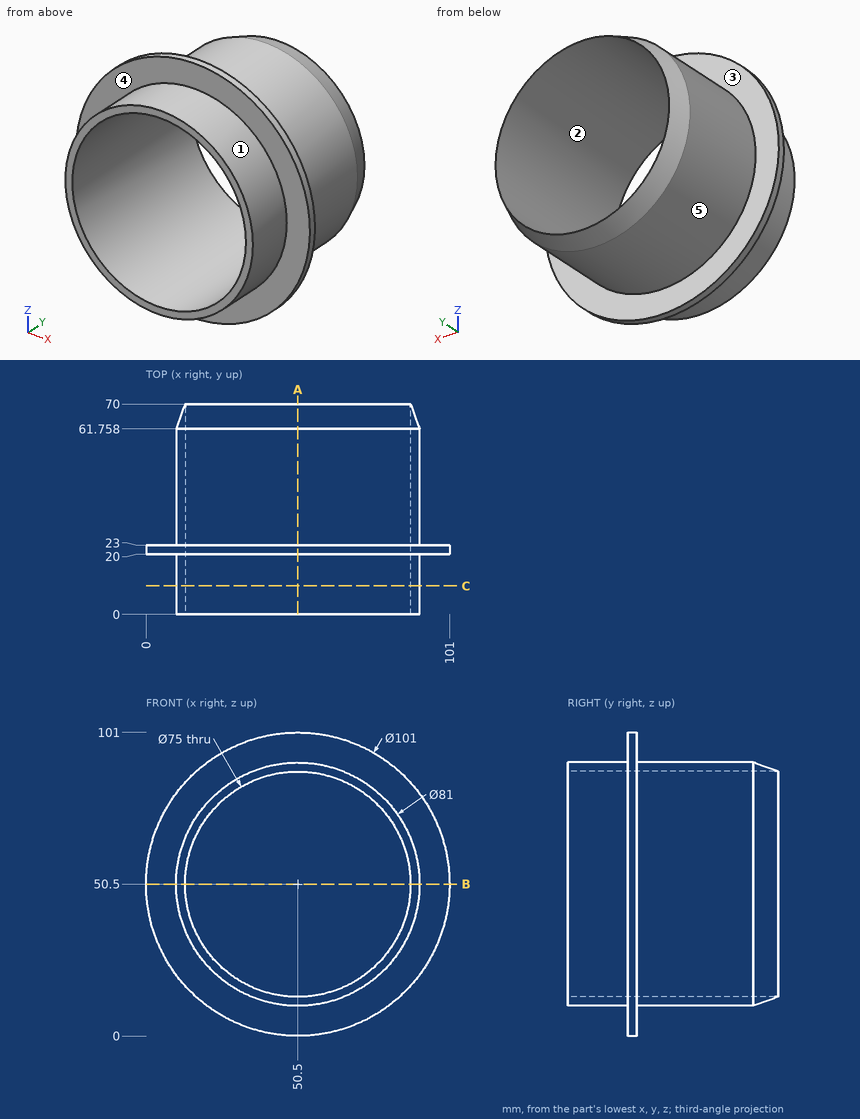
Here's the drawing with two shaded views (mm, measured from the low corner). I have some questions. A direction names the side the tool comes from. Give positions to 0.01 mm unless a question says otherwise; leave off trailing zeros. Loops run counter-clockwise (first coordinate to the right, second up) from the corner with the lowest first, then second, coordinate; pieces in that order, holes last. Notation, with made-up numbers: M -11.75,3.5 L 43.25,3.5 A20 ccw 43.25,16.5 Z; hole C -39,43.5 d1. An arc over 180 degrees is marked long. One line per item, written item: value. Start each with the question number.
1) If I drill on line 1 (Z direction, x = 50.5, y = 14.5); line 2 (X direction, y = 21, z = 50), over which ranges is the centre line in solid material (lowest first)? Write a range as [from, to].
2) If we section it at B-B, the plane z = 50.5: Write out the boundary of the cut face in (x, y).
3) On a 3-axis mill with a long thin cutter (end or side, diameter ignored), from which of +Z, -Z, +X, -X, +Y, -Y can I reach the whole of each face in a straight line? I mean the marked faces 4 and 5. Say none if no direction works.
4) I'm going to push flat-ended pins straight in: pin 1 (12 mm diameter, centred on y = 43.5, z = 64, fed in from -X); pin 2 (4 mm diameter, centred on y = 7.5, z = 30, fed in from -X); pin 3 (1.5 mm diameter, centred on x = 37, y = 7.5, fed in from -Z); pin 4 (12 mm diameter, centred on x = 20.5, z = 80, fed in from -Y). Where does each tip first touch, or does it pass through?
5) If we section it at A-A, the plane x = 50.5: Write out the boundary of the cut face in (y, z).
6) If we section it at C-C, the plane y = 9.5: Write out the boundary of the cut face in (x, z).
7) Thinking about a two-plate mould opening in Z: for the marked faces 1, 2 and 3, which applies, +Z half, -Z half, draft (parallel to the pull), parting line (faces both ways), or undercut?
Completed:
1. line 1: z = [10, 13], [88, 91]
1. line 2: x = [0, 13], [88, 101]
2. outline: M 0,20 L 10,20 L 10,0 L 13,0 L 13,70 L 10,61.76 L 10,23 L 0,23 Z; M 88,0 L 91,0 L 91,20 L 101,20 L 101,23 L 91,23 L 91,61.76 L 88,70 Z
3. face 4: -Y
3. face 5: +Y
4. pin 1: stops at x = 10.7
4. pin 2: stops at x = 14.47
4. pin 3: stops at z = 12.06
4. pin 4: stops at y = 0
5. outline: M 0,10 L 20,10 L 20,0 L 23,0 L 23,10 L 61.76,10 L 70,13 L 0,13 Z; M 0,88 L 70,88 L 61.76,91 L 23,91 L 23,101 L 20,101 L 20,91 L 0,91 Z
6. outline: C 50.5,50.5 d81; hole C 50.5,50.5 d75
7. face 1: parting line
7. face 2: undercut
7. face 3: draft
